Here's how the part is built. I have some questions about the finished solid (model axes, mm). Round coordinates to 2 decimals unless told otherwise and drop trailing zeros. Order: outer loops, then holes, each group sorted by start corner. A loop starts at its lowest first (then second) coordinate and runs counter-clockwise, first axis right, second up. Notation, with made-up numbers: (21.5, 2) -> (80.5, 2) arc R16 cw to (80.5, 29) -> close; hole circle Ø6 at (59.25, 4). An arc over 180 degrees is marked (long way). Answer in a Markdown table with one row per item.
```python
from build123d import *

# Parameters (mm, degrees)
SKETCH1_W           = 114.3
SKETCH1_H           = 177.8
SKETCH1_W_2         = 101.6
SKETCH1_H_2         = 165.1
BOSS_EXTRUDE1_DEPTH = 4.7625
SKETCH2_W           = 12.38677804
SKETCH2_H           = 4.7625
SKETCH2_W_2         = 12.7
BOSS_EXTRUDE2_DEPTH = 4.7625
SKETCH3_W           = 12.7
SKETCH3_H           = 4.7625
BOSS_EXTRUDE3_DEPTH = 4.7625
FILLET1_R           = 2.54
SKETCH5_W           = 114.3
SKETCH5_H           = 12.7
SKETCH5_W_2         = 101.6
SKETCH5_H_2         = 3.81
BOSS_EXTRUDE5_DEPTH = 4.7625
FILLET3_R           = 1.905


with BuildPart() as part:
    # Sketch1 → Boss-Extrude1 (new body)
    with BuildSketch(Plane(origin=(0, 0, 0), x_dir=(1, 0, 0), z_dir=(0, 1, 0))):
        Rectangle(SKETCH1_W, SKETCH1_H)
        Rectangle(SKETCH1_W_2, SKETCH1_H_2, mode=Mode.SUBTRACT)
    extrude(amount=BOSS_EXTRUDE1_DEPTH)

    # Sketch2 → Boss-Extrude2 (add)
    with BuildSketch(Plane.XY.offset(88.9)):
        with Locations((-38.1, 2.38125)):
            Rectangle(SKETCH2_W, SKETCH2_H)
        with Locations((12.7, 2.38125)):
            Rectangle(SKETCH2_W_2, SKETCH2_H)
    extrude(amount=BOSS_EXTRUDE2_DEPTH)

    # Sketch3 → Boss-Extrude3 (add)
    with BuildSketch(Plane(origin=(0, 0, -88.9), x_dir=(-1, 0, 0), z_dir=(0, 0, -1))):
        with Locations((-38.1, 2.38125)):
            Rectangle(SKETCH3_W, SKETCH3_H)
        with Locations((12.7, 2.38125)):
            Rectangle(SKETCH3_W, SKETCH3_H)
    extrude(amount=BOSS_EXTRUDE3_DEPTH)

    # Fillet1
    fillet1_edges = [part.edges().sort_by_distance(p)[0] for p in [
        (50.8, 2.38125, 82.55),
        (50.8, 2.38125, -82.55),
        (-50.8, 2.38125, -82.55),
        (-50.8, 2.38125, 82.55),
    ]]
    fillet(fillet1_edges, radius=FILLET1_R)

    # Sketch5 → Boss-Extrude5 (add)
    with BuildSketch(Plane.XZ):
        Rectangle(SKETCH5_W, SKETCH5_H)
        Rectangle(SKETCH5_W_2, SKETCH5_H_2, mode=Mode.SUBTRACT)
    extrude(amount=-BOSS_EXTRUDE5_DEPTH)

    # Fillet3
    fillet3_edges = [part.edges().sort_by_distance(p)[0] for p in [
        (-50.8, 2.38125, 6.35),
        (-50.8, 2.38125, -6.35),
        (50.8, 2.38125, -6.35),
        (50.8, 2.38125, 6.35),
        (50.8, 2.38125, -1.905),
        (-50.8, 2.38125, -1.905),
        (-50.8, 2.38125, 1.905),
        (50.8, 2.38125, 1.905),
    ]]
    fillet(fillet3_edges, radius=FILLET3_R - 0.0001)  # a hair under: the kernel refuses the full size


solid = part.part
```
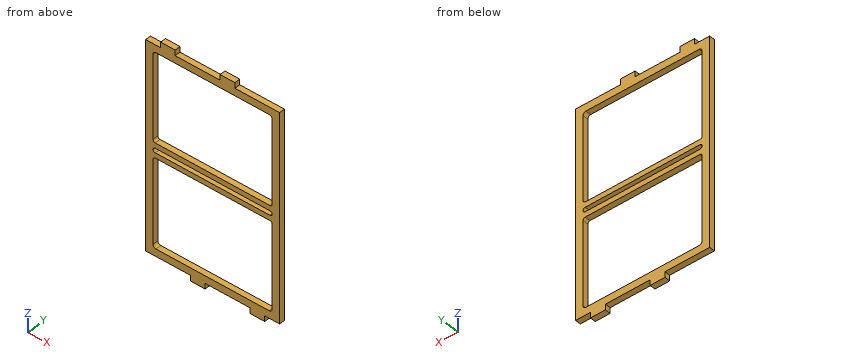
1. Suppose I cut it at A-A on z = 21. Write out the boundary of the cut face in (x, y), then the cut area to 3 significant figures.
Numbers:
| item | result |
|---|---|
| outline | (-57.15, 0) -> (-50.8, 0) -> (-50.8, 4.76) -> (-57.15, 4.76) -> close; (50.8, 0) -> (57.15, 0) -> (57.15, 4.76) -> (50.8, 4.76) -> close |
| area | 60.5 mm2 |
2. Suppose I cut it at B-B on x = -14.5. State how many separate pieces and enclosed holes the cut face has, then the cut area to 3 significant figures.
Numbers:
| item | result |
|---|---|
| separate pieces | 4 |
| enclosed holes | 0 |
| area | 126 mm2 |
3. Please list where these lines run through material, in increasing order: line 1 along Z through (x, y) = (-25, 2.25) (3 decimals); line 2 along X through (y, z) = (2.7, 28); line 3 along Z through (x, y) = (-49.5, 0.8).
Numbers:
| item | result |
|---|---|
| line 1 | z = -88.9 to -82.55, -6.35 to -1.905, 1.905 to 6.35, 82.55 to 88.9 |
| line 2 | x = -57.15 to -50.8, 50.8 to 57.15 |
| line 3 | z = -88.9 to -82.23, -6.45 to -1.81, 1.81 to 6.45, 82.23 to 88.9 |
4. For pin 1 Ø1.4 at (x, y) = (20, 1.5) entering from -Z; pin 2 Ø2.5 at (y, z) = (1.5, -91.5) entering from -X; pin 3 Ø1.4 at (x, y) = (-50, 3) entering from +Z, each with a flat end and sliding along its axis, tell me the tip position at first contact or that it passes through.
Numbers:
| item | result |
|---|---|
| pin 1 | stops at z = -88.9 |
| pin 2 | stops at x = -19.05 |
| pin 3 | stops at z = 88.9 |
